Design review of the part built by this model. Coordinates are the model's own, in mm. A direction names the side the tool comes from. Coordinates: 2 decimals unless noted, no trailing zeros. Loops run counter-clockwise (first coordinate to the right, second up) from the corner with the lowest first, then second, coordinate; pieces in that order, holes last. Notation, with made-up numbers: (41, -4) -> (61, -4) arc R8 ccw to (61, 7) -> close; hole circle Ø1 at (-28, 21). An arc over 180 degrees is marked (long way). Use a Markdown table: item, result. Add a question column.
Q1. For faces 1 (the face through (66.06, 50.62, 6.11)), 2 (the face through (34, 19, 0)), list the 3-axis set-ups (+Z, -Z, +X, -X, +Y, -Y) from which the entire face can be reached by the end or side of a thin tool; tool diameter is ignored.
Q2. For probe 1 along Y at (x, z) = (34, 2); probe 2 along X at (y, z) = (40.5, 6); probe 3 along X at (y, z) = (29.5, 12), list the stretches that pass through material, from the lowest coordinate up.
Q3. Draft analysis for pull direction Z (two halves, no side actions). For faces 3 (the face through (0, 19, 9)), 4 (the face through (73.25, 18.78, 15.91)), 5 (the face through (66.058, 50.622, 13.094)), state which applies: pulls with the +Z half, pulls with the -Z half, needs draft (parallel to the pull), parting line crosses it, or undercut.
Q4. Clearance check with flat-ended pins moving along their axes: pin 1 Ø3 at (y, z) = (55, 6) entering from +X; pin 2 Ø6 at (y, z) = (34, 16.5) entering from -X; pin 3 Ø1 at (y, z) = (16.5, 16) entering from +X. State where each tip first meets the part, or that it passes through.
Q5. Take a section at C-C on x = 13.5. Write out the cut boundary in (y, z), plus the area to 3 significant figures.
Q6. Take a section at B-B on z = 14.25. Write out the cut boundary in (x, y), plus the area to 3 significant figures.
Q7. Take a section at D-D on z = 7.25. Write out the cut boundary in (x, y).
from build123d import *

# Parameters (mm, degrees)
SKETCH1_W           = 76.2
SKETCH1_H           = 38.1
BOSS_EXTRUDE1_DEPTH = 18.542
FILLET1_R           = 9.525
SKETCH2_R           = 2.54
BOSS_EXTRUDE2_DEPTH = 25.4
FILLET2_R           = 2.6035


with BuildPart() as part:
    # Sketch1 → Boss-Extrude1 (new body)
    with BuildSketch(Plane.XY):
        with Locations((38.1, 19.05)):
            Rectangle(SKETCH1_W, SKETCH1_H)
    extrude(amount=BOSS_EXTRUDE1_DEPTH)

    # Fillet1
    # the kernel refuses this fillet: 9.525 mm, written as the material it takes off along each edge
    with BuildSketch(Plane(origin=(76.2, -23.8125, 18.542), x_dir=(0, 0, -1), z_dir=(0, 1, 0))) as fillet1_piece_1:
        with BuildLine():
            CenterArc((FILLET1_R, FILLET1_R), FILLET1_R, 180, 90)
            Line((0, FILLET1_R), (0, 0))
            Line((0, 0), (FILLET1_R, 0))
        make_face()
    extrude(amount=85.725, mode=Mode.SUBTRACT)
    with BuildSketch(Plane(origin=(76.2, -23.8125, 0), x_dir=(0, 0, 1), z_dir=(0, 1, 0))) as fillet1_piece_2:
        with BuildLine():
            CenterArc((FILLET1_R, -FILLET1_R), FILLET1_R, 90, 90)
            Line((0, -FILLET1_R), (0, 0))
            Line((0, 0), (FILLET1_R, 0))
        make_face()
    extrude(amount=85.725, mode=Mode.SUBTRACT)

    # Sketch2 → Boss-Extrude2 (add)
    with BuildSketch(Plane(origin=(0, 38.1, 0), x_dir=(1, 0, 0), z_dir=(0, 1, 0))):
        with Locations(Location((68.576612731, -5.7785, 0), (0, 0, 90))):
            Circle(SKETCH2_R)
        with Locations(Location((68.576612731, -12.7635, 0), (0, 0, 90))):
            Circle(SKETCH2_R)
    extrude(amount=BOSS_EXTRUDE2_DEPTH)

    # Fillet2
    fillet2_edges = [part.edges().sort_by_distance(p)[0] for p in [
        (0, 19.05, 18.542),
        (0, 19.05, 0),
        (0, 38.1, 9.271),
        (0, 0, 9.271),
    ]]
    fillet(fillet2_edges, radius=FILLET2_R)


solid = part.part
Answer list:
| question | item | result |
|---|---|---|
| 1 | face 1 | +Y |
| 1 | face 2 | -Z, +X, -X, +Y, -Y |
| 2 | probe 1 | 0 to 38.1 |
| 2 | probe 2 | 66.05 to 71.11 |
| 2 | probe 3 | 0 to 75.72 |
| 3 | face 3 | needs draft |
| 3 | face 4 | pulls with the +Z half |
| 3 | face 5 | undercut |
| 4 | pin 1 | x = 71.12 |
| 4 | pin 2 | x = 0 |
| 4 | pin 3 | x = 73.65 |
| 5 | outline | (0, 0) -> (38.1, 0) -> (38.1, 18.54) -> (0, 18.54) -> close |
| 5 | area | 706 mm² |
| 6 | outline | (0, 2.6) arc R2.6 ccw to (2.6, 0) -> (74.63, 0) -> (74.63, 38.1) -> (70.64, 38.1) -> (70.64, 63.5) -> (66.52, 63.5) -> (66.52, 38.1) -> (2.6, 38.1) arc R2.6 ccw to (0, 35.5) -> close |
| 6 | area | 2,950 mm² |
| 7 | outline | (0, 2.6) arc R2.6 ccw to (2.6, 0) -> (75.92, 0) -> (75.92, 38.1) -> (70.65, 38.1) -> (70.65, 63.5) -> (66.51, 63.5) -> (66.51, 38.1) -> (2.6, 38.1) arc R2.6 ccw to (0, 35.5) -> close |
